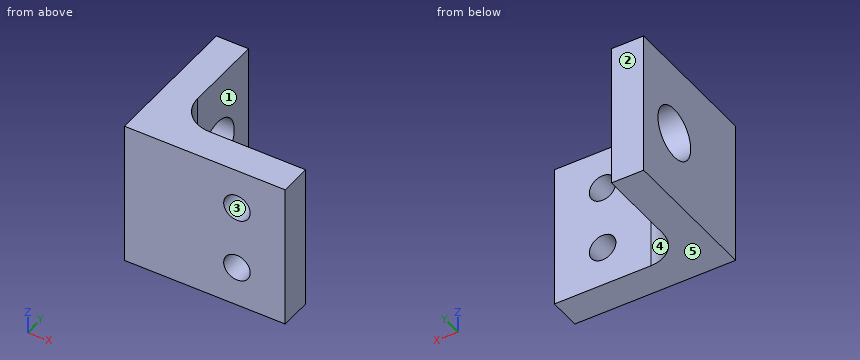
from build123d import *

# Parameters (mm, degrees)
BOSS_EXTRUDE1_DEPTH = 18
SKETCH2_R           = 3.2
CUT_EXTRUDE1_DEPTH  = 25
FILLET1_R           = 4
SKETCH3_R           = 1.65
CUT_EXTRUDE2_DEPTH  = 25


with BuildPart() as part:
    # Sketch1 → Boss-Extrude1 (new body)
    with BuildSketch(Plane.XY):
        Polygon((0, 0), (0, 18), (4, 18), (4, 4), (20, 4), (20, 0), align=None)
    extrude(amount=BOSS_EXTRUDE1_DEPTH)

    # Sketch2 → Cut-Extrude1 (cut)
    with BuildSketch(Plane(origin=(4, 0, 0), x_dir=(0, 0, -1), z_dir=(1, 0, 0))):
        with Locations(Location((-9, 12, 0), (0, 0, 90))):
            Circle(SKETCH2_R)
    extrude(amount=-CUT_EXTRUDE1_DEPTH, mode=Mode.SUBTRACT)

    # Fillet1
    fillet1_edges = [part.edges().sort_by_distance(p)[0] for p in [
        (4, 4, 9),
    ]]
    fillet(fillet1_edges, radius=FILLET1_R)

    # Sketch3 → Cut-Extrude2 (cut)
    with BuildSketch(Plane(origin=(0, 4, 0), x_dir=(1, 0, 0), z_dir=(0, 1, 0))):
        with Locations(Location((14, -5, 0), (0, 0, 180))):
            Circle(SKETCH3_R)
        with Locations(Location((14, -13, 0), (0, 0, 180))):
            Circle(SKETCH3_R)
    extrude(amount=-CUT_EXTRUDE2_DEPTH, mode=Mode.SUBTRACT)


solid = part.part
Geometry: final body of the model. Coordinates: model frame, mm. Face numbers are marked on the shaded views. A direction names the side the tool comes from. Round coordinates to 2 decimals unless told otherwise and drop trailing zeros. Order: outer loops, then holes, each group sorted by start corner. A loop starts at its lowest first (then second) coordinate and runs counter-clockwise, first axis right, second up.
Q1. Section B-B, the plane z = 13. Output: boundary loops of the cut face in (x, y), and give its area (3 significant figures).
Result sheet:
outline: (0, 0) - (12.35, 0) - (12.35, 4) - (8, 4) arc R4 cw to (4, 8) - (4, 18) - (0, 18) - close; (15.65, 0) - (20, 0) - (20, 4) - (15.65, 4) - close
area: 126 mm2
Q2. Pin query (flat end, axial travel): pin 1 (1 mm diameter, centred on y = 12.5, z = 12.5, fed in from +X); pin 2 (4 mm diameter, centred on y = 8.5, z = 10, fed in from +X); pin 3 (9.5 mm diameter, centred on x = 13.5, z = 9, fed in from +Y). Return the tip coordinate at first contact, or that it passes through.
Result sheet:
pin 1: stops at x = 4
pin 2: stops at x = 4.29
pin 3: stops at y = 4
Q3. Section C-C, the plane x = 14. Output: boundary loops of the cut face in (y, z), and give its area (3 significant figures).
Result sheet:
outline: (0, 0) - (4, 0) - (4, 3.35) - (0, 3.35) - close; (0, 6.65) - (4, 6.65) - (4, 11.35) - (0, 11.35) - close; (0, 14.65) - (4, 14.65) - (4, 18) - (0, 18) - close
area: 45.6 mm2
Q4. Material intervals for probe 1 along Z at (x, y) = (14, 2.95); probe 2 along Z at (x, y) = (3.15, 12); probe 3 along Y at (x, z) = (12.25, 14.75), sorted ascending.
Result sheet:
probe 1: z = 0 to 3.35, 6.65 to 11.35, 14.65 to 18
probe 2: z = 0 to 5.8, 12.2 to 18
probe 3: y = 0 to 4
Q5. Section A-A, the plane y = 12. Output: boundary loops of the cut face in (x, z), and give its area (3 significant figures).
Result sheet:
outline: (0, 0) - (4, 0) - (4, 5.8) - (0, 5.8) - close; (0, 12.2) - (4, 12.2) - (4, 18) - (0, 18) - close
area: 46.4 mm2
Q6. Access query for the marked faces 1 and 2. Directions: +Z, -Z, +X, -X, +Y, -Y. A direction counts if a zero-diameter tool reaches every point of the face in a straight line with its end or side. Return the directions, or none.
Result sheet:
face 1: +Z, -Z, +X, +Y
face 2: +Z, -Z, +X, -X, +Y
Q7. Section D-D, the plane y = 2.5. Output: boundary loops of the cut face in (x, z).
Result sheet:
outline: (0, 0) - (20, 0) - (20, 18) - (0, 18) - close; hole circle Ø3.3 at (14, 5); hole circle Ø3.3 at (14, 13)
Q8. Mould query, pull axis X, two halves, no side actions, for the marked faces 3, 4 and 5. Classes: released by +X, released by -X, zero draft, split by the parting line, or undercut.
Result sheet:
face 3: undercut
face 4: released by +X
face 5: zero draft
